Geometry: final body of the model. Coordinates: model frame, mm. A direction names the side the tool comes from. Round coordinates to 2 decimals unless told otherwise and drop trailing zeros. Loops run counter-clockwise (first coordinate to the right, second up) from the corner with the lowest first, then second, coordinate; pieces in that order, holes last. Notation, with made-up numbers: (80.5, -20.75) -> (136.5, -20.75) arc R21 cw to (136.5, 14.25) -> close; hole circle Ø11 at (88, 67.25). An arc over 180 degrees is marked (long way). Answer in a Markdown table with one row per item.
```python
from build123d import *

# Parameters (mm, degrees)
BOSS_EXTRUDE1_DEPTH = 5.715
SKETCH2_W           = 202.5
SKETCH2_H           = 243
CUT_EXTRUDE1_DEPTH  = 6.715


with BuildPart() as part:
    # Model → Boss-Extrude1 (new body)
    with BuildSketch(Plane.XY):
        Polygon((1074.08036017, 22.860238699), (1079.905563672, 22.860238699), (1079.905563672, 28.575245224), (1091.332742073, 28.575245224), (1091.332742073, 22.860238699), (1102.763463785, 22.860238699), (1102.763463785, 28.575245224), (1114.194185497, 28.575245224), (1114.194185497, 22.860238699), (1125.62490721, 22.860238699), (1125.62490721, 28.575245224), (1137.055628922, 28.575245224), (1137.055628922, 22.860238699), (1148.482807323, 22.860238699), (1148.482807323, 28.575245224), (1159.913529035, 28.575245224), (1159.913529035, 22.860238699), (1171.344250747, 22.860238699), (1171.344250747, 28.575245224), (1182.77497246, 28.575245224), (1182.77497246, 22.860238699), (1194.205694172, 22.860238699), (1194.205694172, 28.575245224), (1205.632872573, 28.575245224), (1205.632872573, 22.860238699), (1217.063594285, 22.860238699), (1217.063594285, 28.575245224), (1228.494315997, 28.575245224), (1228.494315997, 22.860238699), (1239.92503771, 22.860238699), (1239.92503771, 28.575245224), (1251.355759422, 28.575245224), (1251.355759422, 22.860238699), (1262.782937823, 22.860238699), (1262.782937823, 28.575245224), (1274.213659535, 28.575245224), (1274.213659535, 22.860238699), (1280.038863036, 22.860238699), (1285.754223893, 22.860238699), (1285.754223893, 28.575245224), (1285.754223893, 288.575408216), (1285.754223893, 294.290414741), (1280.038863036, 294.290414741), (1274.213659535, 294.290414741), (1274.213659535, 288.575408216), (1262.782937823, 288.575408216), (1262.782937823, 294.290414741), (1251.355759422, 294.290414741), (1251.355759422, 288.575408216), (1239.92503771, 288.575408216), (1239.92503771, 294.290414741), (1228.494315997, 294.290414741), (1228.494315997, 288.575408216), (1217.063594285, 288.575408216), (1217.063594285, 294.290414741), (1205.632872573, 294.290414741), (1205.632872573, 288.575408216), (1194.205694172, 288.575408216), (1194.205694172, 294.290414741), (1182.77497246, 294.290414741), (1182.77497246, 288.575408216), (1171.344250747, 288.575408216), (1171.344250747, 294.290414741), (1159.913529035, 294.290414741), (1159.913529035, 288.575408216), (1148.482807323, 288.575408216), (1148.482807323, 294.290414741), (1137.055628922, 294.290414741), (1137.055628922, 288.575408216), (1125.62490721, 288.575408216), (1125.62490721, 294.290414741), (1114.194185497, 294.290414741), (1114.194185497, 288.575408216), (1102.763463785, 288.575408216), (1102.763463785, 294.290414741), (1091.332742073, 294.290414741), (1091.332742073, 288.575408216), (1079.905563672, 288.575408216), (1079.905563672, 294.290414741), (1074.08036017, 294.290414741), (1074.08036017, 288.575408216), (1074.08036017, 28.575245224), align=None)
    extrude(amount=BOSS_EXTRUDE1_DEPTH)

    # Sketch2 → Cut-Extrude1 (cut, through all)
    with BuildSketch(Plane(origin=(0, 0, 0), x_dir=(-1, 0, 0), z_dir=(0, 0, -1))):
        with Locations((-1179.917292032, 158.575323457)):
            Rectangle(SKETCH2_W, SKETCH2_H)
    extrude(amount=-CUT_EXTRUDE1_DEPTH, mode=Mode.SUBTRACT)


solid = part.part
```
Item 1: Pin query (flat end, axial travel): pin 1 Ø1.7 at (x, z) = (1153.5, 2.5) entering from +Y; pin 2 Ø1.7 at (x, z) = (1175.5, 2) entering from -Y. Return the tip coordinate at first contact, or that it passes through.
Answer:
| item | result |
|---|---|
| pin 1 | stops at y = 288.58 |
| pin 2 | stops at y = 28.58 |
Item 2: Cut plane B-B (y = 86). Output: boundary loops of the cut face in (x, z) (3 decimals).
Answer:
| item | result |
|---|---|
| outline | (1074.08, 0) -> (1078.667, 0) -> (1078.667, 5.715) -> (1074.08, 5.715) -> close; (1281.167, 0) -> (1285.754, 0) -> (1285.754, 5.715) -> (1281.167, 5.715) -> close |
Item 3: Reachability of faces 3 (the face through (1077, 22.86, 3)), 4 (the face through (1223, 28.575, 3)), 5 (the face through (1182.775, 291, 3)) from +Z, -Z, +X, -X, +Y, -Y: full face, straight path, thin tool, end or side. Return the list, or none.
Answer:
| item | result |
|---|---|
| face 3 | +Z, -Z, +X, -X, -Y |
| face 4 | +Z, -Z, -Y |
| face 5 | +Z, -Z, +Y |
Item 4: Draft query along X for faces 1 (the face through (1234, 22.86, 3)), 2 (the face through (1194.206, 26, 3)). Return one class per face: pulls with the +X half, pulls with the -X half, needs draft (parallel to the pull), parting line crosses it, or undercut.
Answer:
| item | result |
|---|---|
| face 1 | needs draft |
| face 2 | undercut |
Item 5: Cut plane A-A (x = 1118.5). Output: boundary loops of the cut face in (y, z) (3 decimals).
Answer:
| item | result |
|---|---|
| outline | (22.86, 0) -> (37.075, 0) -> (37.075, 5.715) -> (22.86, 5.715) -> close; (280.075, 0) -> (294.29, 0) -> (294.29, 5.715) -> (280.075, 5.715) -> close |
Item 6: Line query: probe 1 along Y at (x, z) = (1128.5, 4.05); probe 2 along Y at (x, z) = (1139.5, 4.55); probe 3 along X at (y, z) = (113, 5.3). Output: solid intervals per line, ascending. Write a range as [from, to].
Answer:
| item | result |
|---|---|
| probe 1 | y = [28.58, 37.08], [280.08, 288.58] |
| probe 2 | y = [22.86, 37.08], [280.08, 294.29] |
| probe 3 | x = [1074.08, 1078.67], [1281.17, 1285.75] |
